```python
from build123d import *

# Parameters (mm, degrees)
F0_W     = 90
F0_H     = 49.79875
F0_W_2   = 72
F0_H_2   = 39.79875
F0_R     = 3
F1_DEPTH = 3


with BuildPart() as f1:
    # F0 (on Front) → F1 (new body)
    with BuildSketch(Plane.XZ):
        with Locations((0, -0.000125)):
            Rectangle(F0_W, F0_H)
        with Locations((-4, -0.000125)):
            Rectangle(F0_W_2, F0_H_2, mode=Mode.SUBTRACT)
        with Locations((38.5, 5.741427)):
            Circle(F0_R, mode=Mode.SUBTRACT)
        with Locations((38.5, 19.10959)):
            Circle(F0_R, mode=Mode.SUBTRACT)
    extrude(amount=F1_DEPTH)


solid = f1.part
```
CAD build for the part. Positions are in the model's coordinates, mm. A direction names the side the tool comes from. Coordinates: 2 decimals unless noted, no trailing zeros. Write each loop counter-clockwise with the first axis right and the second up, starting at its lowest first coordinate (ties: lowest second). Pieces come first, ordered by that corner, then holes.
(1) Cut at C-C, the plane x = 38.5. List the corners of the cut face in (y, z).
(2) Cut at A-A, the plane z = 10.5. List the corners of the cut face in (x, y).
(3) Drill centre lines: probe 1 along Z at (x, y) = (38.5, -2.15); probe 2 along X at (y, z) = (-1.5, 19); probe 3 along X at (y, z) = (-0.3, -6). Where is each one in solid material? Low to high.
(4) 3-axis set-ups, long thin cutter, end or side, ignore diameter. For faces 4 (the face through (-1, -1, 24.899)), 5 (the face through (-40, -1, 0)): which of +Z, -Z, +X, -X, +Y, -Y reach the whole face in a straight line?
(5) Cut at D-D, the plane y = -2.4. List the corners of the cut face in (x, z).
(6) Two-plate mould, pull along X, no slides. Class faces 1 (the face through (-5, -1, 19.899)), 2 (the face through (45, -1, 0)), 3 (the face through (-1, -1, -24.9)): +X half, -X half, draft (parallel to the pull), parting line (faces both ways), or undercut.
(7) Flat gauge pin, fed straight in: pin 1 (3.5 mm diameter, centred on x = 38.5, z = 19.11, fed in from -Y). Where does the tip first touch, or does it go through?
(8) Cut at B-B, the plane x = 25.5. List the corners of the cut face in (y, z).
Geometry says:
1. outline: (-3, -24.9) - (0, -24.9) - (0, 2.74) - (-3, 2.74) - close; (-3, 8.74) - (0, 8.74) - (0, 16.11) - (-3, 16.11) - close; (-3, 22.11) - (0, 22.11) - (0, 24.9) - (-3, 24.9) - close
2. outline: (-45, -3) - (-40, -3) - (-40, 0) - (-45, 0) - close; (32, -3) - (45, -3) - (45, 0) - (32, 0) - close
3. probe 1: z = -24.9 to 2.74, 8.74 to 16.11, 22.11 to 24.9
3. probe 2: x = -45 to -40, 32 to 35.5, 41.5 to 45
3. probe 3: x = -45 to -40, 32 to 45
4. face 4: +Z, +X, -X, +Y, -Y
4. face 5: +Y, -Y
5. outline: (-45, -24.9) - (45, -24.9) - (45, 24.9) - (-45, 24.9) - close; hole (-40, -19.9) - (32, -19.9) - (32, 19.9) - (-40, 19.9) - close; hole circle Ø6 at (38.5, 5.74); hole circle Ø6 at (38.5, 19.11)
6. face 1: undercut
6. face 2: +X half
6. face 3: draft
7. pin 1: passes through
8. outline: (-3, -24.9) - (0, -24.9) - (0, -19.9) - (-3, -19.9) - close; (-3, 19.9) - (0, 19.9) - (0, 24.9) - (-3, 24.9) - close
